```python
from build123d import *

# Parameters (mm, degrees)
SKETCH1_R          = 8.25
BASE_EXTRUDE_DEPTH = 8


with BuildPart() as part:
    # Sketch1 → Base-Extrude (new body)
    with BuildSketch(Plane.XY):
        with BuildLine():
            Line((45, 14.798648587), (45, -14.798648587))
            ThreePointArc((45, -14.798648587), (44.800644447, -16.785447123), (44.210526316, -18.693029794))
            ThreePointArc((44.210526316, -18.693029794), (33.941125497, -33.941125497), (18.693029794, -44.210526316))
            ThreePointArc((18.693029794, -44.210526316), (16.785447123, -44.800644447), (14.798648587, -45))
            Line((14.798648587, -45), (-14.798648587, -45))
            ThreePointArc((-14.798648587, -45), (-16.785447123, -44.800644447), (-18.693029794, -44.210526316))
            ThreePointArc((-18.693029794, -44.210526316), (-23.05203941, -42.102297788), (-27.176470588, -39.565634664))
            ThreePointArc((-27.176470588, -39.565634664), (-54.625644624, -26.342588675), (-84.782545805, -21.998925285))
            ThreePointArc((-84.782545805, -21.998925285), (-100.479276593, -15.633041807), (-107, 0))
            ThreePointArc((-107, 0), (-100.479276593, 15.633041807), (-84.782545805, 21.998925285))
            ThreePointArc((-84.782545805, 21.998925285), (-54.625644624, 26.342588675), (-27.176470588, 39.565634664))
            ThreePointArc((-27.176470588, 39.565634664), (-23.05203941, 42.102297788), (-18.693029794, 44.210526316))
            ThreePointArc((-18.693029794, 44.210526316), (-16.785447123, 44.800644447), (-14.798648587, 45))
            Line((-14.798648587, 45), (14.798648587, 45))
            ThreePointArc((14.798648587, 45), (16.785447123, 44.800644447), (18.693029794, 44.210526316))
            ThreePointArc((18.693029794, 44.210526316), (33.941125497, 33.941125497), (44.210526316, 18.693029794))
            ThreePointArc((44.210526316, 18.693029794), (44.800644447, 16.785447123), (45, 14.798648587))
        make_face()
        with Locations((-85, 0)):
            Circle(SKETCH1_R, mode=Mode.SUBTRACT)
        Circle(SKETCH1_R, mode=Mode.SUBTRACT)
        with BuildLine():
            Line((-9.9, 27.819597409), (-9.9, 17.433588271))
            ThreePointArc((-9.9, 17.433588271), (-9.965213375, 17.186686284), (-10.143842365, 17.004189545))
            ThreePointArc((-10.143842365, 17.004189545), (-14.000714267, 14.000714267), (-17.004189545, 10.143842365))
            ThreePointArc((-17.004189545, 10.143842365), (-17.186686284, 9.965213375), (-17.433588271, 9.9))
            Line((-17.433588271, 9.9), (-27.819597409, 9.9))
            ThreePointArc((-27.819597409, 9.9), (-28.23041494, 10.114993059), (-28.2879408, 10.575084175))
            ThreePointArc((-28.2879408, 10.575084175), (-21.354624792, 21.354624792), (-10.575084175, 28.2879408))
            ThreePointArc((-10.575084175, 28.2879408), (-10.114993059, 28.23041494), (-9.9, 27.819597409))
        make_face(mode=Mode.SUBTRACT)
        with BuildLine():
            Line((17.433588271, 9.9), (27.819597409, 9.9))
            ThreePointArc((27.819597409, 9.9), (28.23041494, 10.114993059), (28.2879408, 10.575084175))
            ThreePointArc((28.2879408, 10.575084175), (21.354624792, 21.354624792), (10.575084175, 28.2879408))
            ThreePointArc((10.575084175, 28.2879408), (10.114993059, 28.23041494), (9.9, 27.819597409))
            Line((9.9, 27.819597409), (9.9, 17.433588271))
            ThreePointArc((9.9, 17.433588271), (9.965213375, 17.186686284), (10.143842365, 17.004189545))
            ThreePointArc((10.143842365, 17.004189545), (14.000714267, 14.000714267), (17.004189545, 10.143842365))
            ThreePointArc((17.004189545, 10.143842365), (17.186686284, 9.965213375), (17.433588271, 9.9))
        make_face(mode=Mode.SUBTRACT)
        with BuildLine():
            Line((9.9, -27.819597409), (9.9, -17.433588271))
            ThreePointArc((9.9, -17.433588271), (9.965213375, -17.186686284), (10.143842365, -17.004189545))
            ThreePointArc((10.143842365, -17.004189545), (14.000714267, -14.000714267), (17.004189545, -10.143842365))
            ThreePointArc((17.004189545, -10.143842365), (17.186686284, -9.965213375), (17.433588271, -9.9))
            Line((17.433588271, -9.9), (27.819597409, -9.9))
            ThreePointArc((27.819597409, -9.9), (28.23041494, -10.114993059), (28.2879408, -10.575084175))
            ThreePointArc((28.2879408, -10.575084175), (21.354624792, -21.354624792), (10.575084175, -28.2879408))
            ThreePointArc((10.575084175, -28.2879408), (10.114993059, -28.23041494), (9.9, -27.819597409))
        make_face(mode=Mode.SUBTRACT)
        with BuildLine():
            Line((-17.433588271, -9.9), (-27.819597409, -9.9))
            ThreePointArc((-27.819597409, -9.9), (-28.23041494, -10.114993059), (-28.2879408, -10.575084175))
            ThreePointArc((-28.2879408, -10.575084175), (-21.354624792, -21.354624792), (-10.575084175, -28.2879408))
            ThreePointArc((-10.575084175, -28.2879408), (-10.114993059, -28.23041494), (-9.9, -27.819597409))
            Line((-9.9, -27.819597409), (-9.9, -17.433588271))
            ThreePointArc((-9.9, -17.433588271), (-9.965213375, -17.186686284), (-10.143842365, -17.004189545))
            ThreePointArc((-10.143842365, -17.004189545), (-14.000714267, -14.000714267), (-17.004189545, -10.143842365))
            ThreePointArc((-17.004189545, -10.143842365), (-17.186686284, -9.965213375), (-17.433588271, -9.9))
        make_face(mode=Mode.SUBTRACT)
    extrude(amount=BASE_EXTRUDE_DEPTH)


solid = part.part
```
Part model, mm, in its own coordinate system. A direction names the side the tool comes from. Give positions to 0.01 mm unless a question says otherwise; leave off trailing zeros. Order: outer loops, then holes, each group sorted by start corner. A loop starts at its lowest first (then second) coordinate and runs counter-clockwise, first axis right, second up. Notation, with made-up numbers: (88.5, 14) - (108.5, 14) arc R29 cw to (108.5, 40) - close; hole circle Ø11 at (-1, 67.25). An arc over 180 degrees is marked (long way). Use one line per item in the form item = value.
Item 1: Slice it at C-C on y = 35. Give the cut face in (x, z), and give its area (3 significant figures).
Solution:
outline = (-34.48, 0) - (32.85, 0) - (32.85, 8) - (-34.48, 8) - close
area = 539 mm2
Item 2: Pin check, flat tips, straight feed: pin 1 Ø2 at (x, z) = (-28.5, 3) entering from -Y; pin 2 Ø4 at (y, z) = (-22, 5.5) entering from +X; pin 3 Ø1 at (x, z) = (21, 2) entering from +Y. Stop position of each tip, or through.
Solution:
pin_1 = -39.34
pin_2 = 43.63
pin_3 = 43.4
Item 3: Which spindle directions (+Z, -Z, +X, -X, +Y, -Y) get a long thin tool onto all of the face, cutting with end or side? Do faces 1 (the face through (44.795, 16.813, 3.944)), 2 (the face through (9.9, -23, 4)). Say none if no direction does.
Solution:
face_1 = +Z, -Z, +X, +Y
face_2 = +Z, -Z
Item 4: Two-plate mould, pull along Y, no slides. Class faces 3 (the face through (-23.11, 42.07, 3.94)), 4 (the face through (21.48, 21.23, 3.94)), 5 (the face through (44.806, -16.758, 3.944)): released by +Y, released by -Y, zero draft, split by the parting line, or undercut.
Solution:
face_3 = released by +Y
face_4 = undercut
face_5 = released by -Y
Item 5: Probe probe 1 along Y at (x, z) = (0, 2.5); probe 2 along Y at (x, z) = (-85, 4); probe 3 along X at (y, z) = (18, 5.75). List the from-to ranges inside material, lowest first. Write a range as from..to.
Solution:
probe_1 = -45..-8.25, 8.25..45
probe_2 = -22..-8.25, 8.25..22
probe_3 = -97.65..-24.25, -9.9..9.9, 24.25..44.47
Item 6: Slice it at A-A on x = 0. Give the cut face in (y, z), and give its area (3 significant figures).
Solution:
outline = (-45, 0) - (-8.25, 0) - (-8.25, 8) - (-45, 8) - close; (8.25, 0) - (45, 0) - (45, 8) - (8.25, 8) - close
area = 588 mm2
Item 7: Slice it at D-D on x = -56. Give the cut face in (y, z).
Solution:
outline = (-25.93, 0) - (25.93, 0) - (25.93, 8) - (-25.93, 8) - close
Item 8: Slice it at B-B on z = 4.5. Count the separate pieces of the cut face and the enclosed holes in it, and give its area (3 significant figures).
Solution:
separate_pieces = 1
enclosed_holes = 6
area = 8,610 mm2
